```python
from build123d import *

# Parameters (mm, degrees)
SKETCH1_R   = 20
SKETCH1_R_2 = 1.1303
SKETCH1_R_3 = 0.75
SKETCH1_R_4 = 0.635
PCB_DEPTH   = 0.6


with BuildPart() as part:
    # Sketch1 → PCB (new body)
    with BuildSketch(Plane(origin=(0, 0, 0), x_dir=(1, 0, 0), z_dir=(0, 1, 0))):
        with Locations(Location((0, 0, 0), (0, 0, 270))):
            Circle(SKETCH1_R)
        with Locations(Location((0, 0, 0), (0, 0, 270))):
            Circle(SKETCH1_R_2, mode=Mode.SUBTRACT)
        with Locations(Location((1.5, 5, 0), (0, 0, 270))):
            Circle(SKETCH1_R_3, mode=Mode.SUBTRACT)
        with Locations(Location((-1.5, -5, 0), (0, 0, 270))):
            Circle(SKETCH1_R_3, mode=Mode.SUBTRACT)
        with Locations(Location((2.05801875, 12.846715625, 0), (0, 0, 270))):
            Circle(SKETCH1_R_4, mode=Mode.SUBTRACT)
        with Locations(Location((-2.05801875, -12.846715625, 0), (0, 0, 270))):
            Circle(SKETCH1_R_4, mode=Mode.SUBTRACT)
    extrude(amount=PCB_DEPTH)


solid = part.part
```
Check sheet for the modelled part. Datum: model origin and axes. Units: mm. Coordinates: 2 decimals unless noted, no trailing zeros. Loops run counter-clockwise (first coordinate to the right, second up) from the corner with the lowest first, then second, coordinate; pieces in that order, holes last.
1) Sectioned sample at A-A (z = 0). Record the boundary of the cut face in (x, y).
2) Sectioned sample at B-B (x = 0). Record the boundary of the cut face in (y, z).
3) Sectioned sample at C-C (y = 0.35). Record the boundary of the cut face in (x, z) (3 decimals).
4) Sectioned sample at D-D (x = -15.5). Record the boundary of the cut face in (y, z), and give its area (3 significant figures).
5) Release check for a two-part mould opening along Z. For faces 1 (the face through (-19.524, 0.296, -4.336)), 2 (the face through (-0.99, 0.3, 4.45)), 3 (the face through (0, 0, 4)) record: released by +Z, released by -Z, zero draft, split by the parting line, or undercut.
6) Gauge pin test, flat end, axial feed: pin 1 (1.2 mm diameter, centred on x = 1.5, z = -5, fed in from +Y). Record the tip position at first contact, or that the pin passes through.
7) Material ranges on probe 1 along X at (y, z) = (0.4, 0); probe 2 along Z at (x, y) = (-1, 0.1); probe 3 along X at (y, z) = (0.4, 5), recorded low to high.
Check sheet entries:
1. outline: (-20, 0) - (-1.13, 0) - (-1.13, 0.6) - (-20, 0.6) - close; (1.13, 0) - (20, 0) - (20, 0.6) - (1.13, 0.6) - close
2. outline: (0, -20) - (0.6, -20) - (0.6, -1.13) - (0, -1.13) - close; (0, 1.13) - (0.6, 1.13) - (0.6, 20) - (0, 20) - close
3. outline: circle Ø40 at (0, 0); hole circle Ø1.27 at (-2.058, 12.847); hole circle Ø1.5 at (-1.5, 5); hole circle Ø2.261 at (0, 0); hole circle Ø1.5 at (1.5, -5); hole circle Ø1.27 at (2.058, -12.847)
4. outline: (0, -12.64) - (0.6, -12.64) - (0.6, 12.64) - (0, 12.64) - close
4. area: 15.2 mm2
5. face 1: split by the parting line
5. face 2: undercut
5. face 3: zero draft
6. pin 1: passes through
7. probe 1: x = -20 to -1.13, 1.13 to 20
7. probe 2: z = -19.97 to -0.53, 0.53 to 4.44, 5.56 to 19.97
7. probe 3: x = -19.36 to -2.25, -0.75 to 19.36
